from build123d import *

# Parameters (mm, degrees)
SKETCH1_W           = 200
SKETCH1_H           = 30
BOSS_EXTRUDE1_DEPTH = 3
SKETCH2_W           = 20.5
SKETCH2_H           = 20.5
CUT_EXTRUDE1_DEPTH  = 3
SKETCH3_W           = 30
SKETCH3_H           = 30
SKETCH3_W_2         = 20.5
SKETCH3_H_2         = 20.5
BOSS_EXTRUDE2_DEPTH = 20
CHAMFER1_SIZE       = 3
SKETCH4_R           = 1.65
CUT_EXTRUDE2_DEPTH  = 40
CHAMFER2_SIZE       = 3
CUT_EXTRUDE3_DEPTH  = 40
SKETCH6_W           = 50
SKETCH6_H           = 2
BOSS_EXTRUDE3_DEPTH = 17
CUT_EXTRUDE4_DEPTH  = 17
SKETCH8_R           = 3.302
CUT_EXTRUDE5_DEPTH  = 17
SKETCH9_R           = 3.302
CUT_EXTRUDE6_DEPTH  = 17
SKETCH10_R          = 6.5
CUT_EXTRUDE7_DEPTH  = 1
SKETCH11_R          = 6.5
CUT_EXTRUDE8_DEPTH  = 1
FILLET1_R           = 5


with BuildPart() as part:
    # Sketch1 → Boss-Extrude1 (new body)
    with BuildSketch(Plane(origin=(0, 0, 0), x_dir=(1, 0, 0), z_dir=(0, 1, 0))):
        Rectangle(SKETCH1_W, SKETCH1_H)
    extrude(amount=BOSS_EXTRUDE1_DEPTH)

    # Sketch2 → Cut-Extrude1 (cut)
    with BuildSketch(Plane(origin=(0, 3, 0), x_dir=(1, 0, 0), z_dir=(0, 1, 0))):
        Rectangle(SKETCH2_W, SKETCH2_H)
    extrude(amount=-CUT_EXTRUDE1_DEPTH, mode=Mode.SUBTRACT)

    # Sketch3 → Boss-Extrude2 (add)
    with BuildSketch(Plane(origin=(0, 3, 0), x_dir=(1, 0, 0), z_dir=(0, 1, 0))):
        Rectangle(SKETCH3_W, SKETCH3_H)
        Rectangle(SKETCH3_W_2, SKETCH3_H_2, mode=Mode.SUBTRACT)
    extrude(amount=BOSS_EXTRUDE2_DEPTH)

    # Chamfer1
    chamfer1_edges = [part.edges().sort_by_distance(p)[0] for p in [
        (15, 13, 15),
        (15, 13, -15),
        (-15, 13, -15),
        (-15, 13, 15),
    ]]
    chamfer(chamfer1_edges, length=CHAMFER1_SIZE)

    # Sketch4 → Cut-Extrude2 (cut)
    with BuildSketch(Plane.XY.offset(15)):
        with Locations((0, 13.514664597)):
            Circle(SKETCH4_R)
    extrude(amount=-CUT_EXTRUDE2_DEPTH, mode=Mode.SUBTRACT)

    # Chamfer2
    # the kernel refuses this chamfer: 3 mm, written as the material it takes off along each edge
    with BuildSketch(Plane(origin=(19.715048964, 23, -15), x_dir=(0, -0.9996219169112968, -0.02749587661058619), z_dir=(-1, 0, 0))) as chamfer2_piece_1:
        Polygon((CHAMFER2_SIZE * 0.999621916911, CHAMFER2_SIZE * 0.0274958766106), (-CHAMFER2_SIZE * 0.0274958766106, CHAMFER2_SIZE * 0.999621916911), (0, 0), align=None)
    extrude(amount=39.430097928, mode=Mode.SUBTRACT)
    with BuildSketch(Plane(origin=(15, 23, 19.715048964), x_dir=(-0.9996219169112968, 0.02749587661058678, 0), z_dir=(0, 0, -1)), Plane(origin=(-19.715048964, 23, 15), x_dir=(0, 0.02749587661058678, -0.9996219169112968), z_dir=(1, 0, 0)), Plane(origin=(-15, 23, -19.715048964), x_dir=(0.9996219169112968, 0.02749587661058678, 0), z_dir=(0, 0, 1))) as chamfer2_piece_2:
        Polygon((CHAMFER2_SIZE * 0.999621916911, -CHAMFER2_SIZE * 0.0274958766106), (-CHAMFER2_SIZE * 0.0274958766106, -CHAMFER2_SIZE * 0.999621916911), (0, 0), align=None)
    extrude(amount=39.430097928, mode=Mode.SUBTRACT)

    # Sketch5 → Cut-Extrude3 (cut)
    with BuildSketch(Plane(origin=(0, 3, 0), x_dir=(1, 0, 0), z_dir=(0, 1, 0))):
        Polygon((-12, 15), (-100, 8), (-100, 15), align=None)
        Polygon((-12, -15), (-100, -15), (-100, -8), align=None)
        Polygon((12, 15), (100, 15), (100, 8), align=None)
        Polygon((12, -15), (100, -15), (100, -8), align=None)
    extrude(amount=-CUT_EXTRUDE3_DEPTH, mode=Mode.SUBTRACT)

    # Sketch6 → Boss-Extrude3 (add)
    with BuildSketch(Plane(origin=(0, 3, 0), x_dir=(1, 0, 0), z_dir=(0, 1, 0))):
        with Locations((-40, -0.368394866)):
            Rectangle(SKETCH6_W, SKETCH6_H)
        with Locations((40, -0.368394866)):
            Rectangle(SKETCH6_W, SKETCH6_H)
    extrude(amount=BOSS_EXTRUDE3_DEPTH)

    # Sketch7 → Cut-Extrude4 (cut)
    with BuildSketch(Plane.XY.offset(1.368394866)):
        Polygon((-15, 20), (-65, 3), (-71.38859119, 29.520775186), align=None)
        Polygon((15, 20), (65, 3), (84.413316585, 43.135600108), align=None)
    extrude(amount=-CUT_EXTRUDE4_DEPTH, mode=Mode.SUBTRACT)

    # Sketch8 → Cut-Extrude5 (cut)
    with BuildSketch(Plane.XY.offset(1.368394866)):
        with Locations((-30, 8.659349902)):
            Circle(SKETCH8_R)
        with Locations((30, 8.659349902)):
            Circle(SKETCH8_R)
    extrude(amount=-CUT_EXTRUDE5_DEPTH, mode=Mode.SUBTRACT)

    # Sketch9 → Cut-Extrude6 (cut)
    with BuildSketch(Plane(origin=(0, 3, 0), x_dir=(1, 0, 0), z_dir=(0, 1, 0))):
        with Locations(Location((-90, 0, 0), (0, 0, 270))):
            Circle(SKETCH9_R)
        with Locations(Location((90, 0, 0), (0, 0, 270))):
            Circle(SKETCH9_R)
    extrude(amount=-CUT_EXTRUDE6_DEPTH, mode=Mode.SUBTRACT)

    # Sketch10 → Cut-Extrude7 (cut)
    with BuildSketch(Plane(origin=(0, 3, 0), x_dir=(1, 0, 0), z_dir=(0, 1, 0))):
        with Locations(Location((90, 0, 0), (0, 0, 270))):
            Circle(SKETCH10_R)
    extrude(amount=-CUT_EXTRUDE7_DEPTH, mode=Mode.SUBTRACT)

    # Sketch11 → Cut-Extrude8 (cut)
    with BuildSketch(Plane(origin=(0, 3, 0), x_dir=(1, 0, 0), z_dir=(0, 1, 0))):
        with Locations(Location((-90, 0, 0), (0, 0, 270))):
            Circle(SKETCH11_R)
    extrude(amount=-CUT_EXTRUDE8_DEPTH, mode=Mode.SUBTRACT)

    # Fillet1
    fillet1_edges = [part.edges().sort_by_distance(p)[0] for p in [
        (-100, 1.5, -8),
        (-100, 1.5, 8),
        (100, 1.5, -8),
        (100, 1.5, 8),
    ]]
    fillet(fillet1_edges, radius=FILLET1_R)


solid = part.part
Verification items for the finished model (mm, model axes). A direction names the side the tool comes from. Coordinates: 2 decimals unless noted, no trailing zeros. Write each loop counter-clockwise with the first axis right and the second up, starting at its lowest first coordinate (ties: lowest second). Pieces come first, ordered by that corner, then holes. Notation, with made-up numbers: M 54.25,-21 L 58.25,-21 A24 ccw 58.25,11 Z; hole C 8.5,16 d9. An arc over 180 degrees is marked long. Use a Markdown table: item, result.
Q1. Draft check along Z on faces 1 (the face through (34, 9, -0.632)), 2 (the face through (-98.64, 1.48, 6.81)), 3 (the face through (15, 11, 7)), 4 (the face through (-96.345, 2.507, -1.409)). Enter one of: +Z half, -Z half, draft (parallel to the pull), parting line (faces both ways), or undercut.
Reply:
| item | result |
|---|---|
| face 1 | -Z half |
| face 2 | +Z half |
| face 3 | draft |
| face 4 | undercut |
Q2. Sectioned sample at B-B, the plane x = -30. Record the boundary of the cut face in (y, z).
Reply:
| item | result |
|---|---|
| outline | M 0,-13.57 L 3,-13.57 L 3,-0.63 L 5.36,-0.63 L 5.36,1.37 L 3,1.37 L 3,13.57 L 0,13.57 Z; M 11.96,-0.63 L 14.9,-0.63 L 14.9,1.37 L 11.96,1.37 Z |
Q3. Sectioned sample at A-A, the plane x = 0. Record the boundary of the cut face in (y, z), plus the area to 3 significant figures.
Reply:
| item | result |
|---|---|
| outline | M 0,-15 L 11.86,-15 L 11.86,-10.25 L 0,-10.25 Z; M 0,10.25 L 11.86,10.25 L 11.86,15 L 0,15 Z; M 15.16,-15 L 20,-15 L 23,-12 L 23,-10.25 L 15.16,-10.25 Z; M 15.16,10.25 L 23,10.25 L 23,12 L 20,15 L 15.16,15 Z |
| area | 178 mm² |
Q4. Sectioned sample at D-D, the plane x = 90. Record the boundary of the cut face in (y, z), plus the area to 3 significant figures.
Reply:
| item | result |
|---|---|
| outline | M 0,-8.8 L 3,-8.8 L 3,-6.5 L 2,-6.5 L 2,-3.3 L 0,-3.3 Z; M 0,3.3 L 2,3.3 L 2,6.5 L 3,6.5 L 3,8.8 L 0,8.8 Z |
| area | 26.6 mm² |
Q5. Go/stop test with flat-tipped pins: P1, Ø5, axis at y = 17, z = -10, coming from the +X side; P2, Ø5, axis at x = 62, z = 8, coming from the +Y side; P3, Ø4, axis at x = -30, y = 8.66, coming from the +Z side; P4, Ø10.5, axis at x = 30, y = 8.66, coming from the -Z side. Record where each tip stops, or that it passes through.
Reply:
| item | result |
|---|---|
| P1 | stops at x = 15 |
| P2 | stops at y = 3 |
| P3 | passes through |
| P4 | stops at z = -0.63 |
Q6. Thickness scan on line 1 (X direction, y = 2.4, z = 0); line 2 (X direction, y = 1, z = 0); line 3 (X direction, y = 14.5, z = 9). Record the ranges inside material, lowest first.
Reply:
| item | result |
|---|---|
| line 1 | x = -100 to -96.5, -83.5 to -10.25, 10.25 to 83.5, 96.5 to 100 |
| line 2 | x = -100 to -93.3, -86.7 to -10.25, 10.25 to 86.7, 93.3 to 100 |
| line 3 | x = -15 to -10.25, 10.25 to 15 |
Q7. Sectioned sample at C-C, the plane x = 50.5. Record the boundary of the cut face in (y, z), plus the area to 3 significant figures.
Reply:
| item | result |
|---|---|
| outline | M 0,-11.94 L 3,-11.94 L 3,-0.63 L 7.93,-0.63 L 7.93,1.37 L 3,1.37 L 3,11.94 L 0,11.94 Z |
| area | 81.5 mm² |
Q8. Set-up check for faces 5 (the face through (-35, 8, -0.632)), 6 (the face through (-15, 11, 7)), 7 (the face through (-47, 3, 3)), 8 (the face through (0, 11, 10.25)), 9 (the face through (34, 9, 1.368)): record each of +Z, -Z, +X, -X, +Y, -Y from which the full face is reachable in a straight line by a thin tool's end or side.
Reply:
| item | result |
|---|---|
| face 5 | -Z, -X, +Y |
| face 6 | +Z, -X, +Y |
| face 7 | -X, +Y |
| face 8 | +Y, -Y |
| face 9 | +Z, +X, +Y |
